Build history of the part. All positions in model axes, mm. Round coordinates to 2 decimals unless told otherwise and drop trailing zeros. Loops run counter-clockwise (first coordinate to the right, second up) from the corner with the lowest first, then second, coordinate; pieces in that order, holes last. Notation, with made-up numbers: M 42,41.25 L 89,41.25 A12 cw 89,60.25 Z; hole C -25,27 d1. An arc over 180 degrees is marked long. Write each question's results on one line, items separated by ' | '. Start each with the question number.
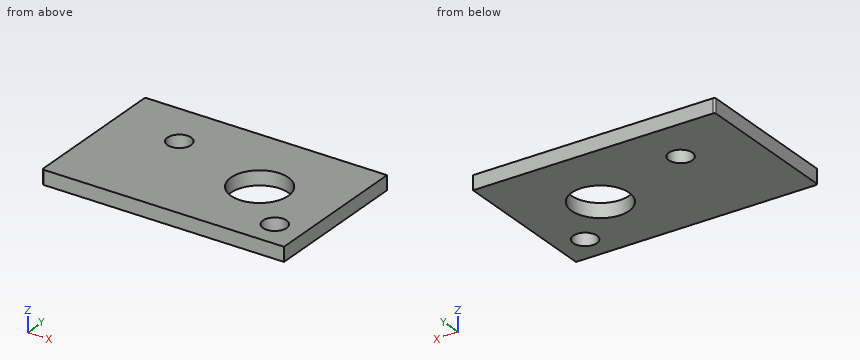
```python
from build123d import *

# Parameters (mm, degrees)
SKETCH1_R          = 1.25
SKETCH1_R_2        = 3.025
BASE_FLANGE1_DEPTH = 1.5


# Sheet-metal steps are written as plain solids
with BuildPart() as part:
    # Sketch1 → Base-Flange1 (new body)
    with BuildSketch(Plane.XY):
        with BuildLine():
            Line((0, 16), (-25.3, 16))
            ThreePointArc((-25.3, 16), (-25.441421356, 15.941421356), (-25.5, 15.8))
            Line((-25.5, 15.8), (-25.5, 0.2))
            ThreePointArc((-25.5, 0.2), (-25.441421356, 0.058578644), (-25.3, 0))
            Line((-25.3, 0), (0, 0))
            Line((0, 0), (0, 16))
        make_face()
        with Locations((-3, 3)):
            Circle(SKETCH1_R, mode=Mode.SUBTRACT)
        with Locations((-8, 8)):
            Circle(SKETCH1_R_2, mode=Mode.SUBTRACT)
        with Locations((-18.5, 11)):
            Circle(SKETCH1_R, mode=Mode.SUBTRACT)
    extrude(amount=-BASE_FLANGE1_DEPTH)


solid = part.part
```
Item 1: Saw through at B-B, the plane z = -1.25. Give the cut face in (x, y) (3 decimals).
Item 2: Drop a flat-ended pin along its axis: pin 1 (1 mm diameter, centred on x = -7.5, y = 7.5, fed in from -Z). Give the stop position or say it passes through.
Item 3: Saw through at C-C, the plane y = 3. Give the cut face in (x, z), then the cut area to 3 significant figures.
Item 4: Drill centre lines: line 1 along Y through (x, z) = (-3, -0.9); line 2 along Y through (x, z) = (-18.5, -0.4); line 3 along X through (y, z) = (5.25, -0.45). Where is each one in solid material? Low to high. Write a range as [from, to].
Item 5: Saw through at A-A, the plane x = -8. Give the cut face in (y, z) (3 decimals).
Working result:
1) outline: M -25.5,0.2 A0.2 ccw -25.3,0 L 0,0 L 0,16 L -25.3,16 A0.2 ccw -25.5,15.8 Z; hole C -18.5,11 d2.5; hole C -8,8 d6.05; hole C -3,3 d2.5
2) pin 1: passes through
3) outline: M -25.5,-1.5 L -4.25,-1.5 L -4.25,0 L -25.5,0 Z; M -1.75,-1.5 L 0,-1.5 L 0,0 L -1.75,0 Z | area: 34.5 mm²
4) line 1: y = [0, 1.75], [4.25, 16] | line 2: y = [0, 9.75], [12.25, 16] | line 3: x = [-25.5, -9.26], [-6.74, 0]
5) outline: M 0,-1.5 L 4.975,-1.5 L 4.975,0 L 0,0 Z; M 11.025,-1.5 L 16,-1.5 L 16,0 L 11.025,0 Z
